```python
from build123d import *

# Parameters (mm, degrees)
F_1P5MM_64_START              = -32
F_1P5MM_64_DEPTH              = 64
CUT_EXTRUDE_M3_1_DEPTH        = 100
CUT_EXTRUDE_M3_1_DEPTH_BACK   = 100
SKETCH_2_R                    = 1.65
CUT_EXTRUDE_M3_1_2_DEPTH      = 100
CUT_EXTRUDE_M3_1_2_DEPTH_BACK = 100
SKETCH_3_R                    = 1.65
CUT_EXTRUDE_M3_1_3_DEPTH      = 100
CUT_EXTRUDE_M3_1_3_DEPTH_BACK = 100
SKETCH_4_R                    = 1.65
CUT_EXTRUDE_M3_1_4_DEPTH      = 100
CUT_EXTRUDE_M3_1_4_DEPTH_BACK = 100
SKETCH_5_R                    = 1.65


with BuildPart() as part:
    # 草图1 → 1p5mm铝合金直角座_宽64 (new body)
    with BuildSketch(Plane.XY.offset(F_1P5MM_64_START)):
        Polygon((0, 0), (16, 0), (16, 1.5), (1.5, 1.5), (1.5, 14), (0, 14), align=None)
    extrude(amount=F_1P5MM_64_DEPTH)

    # 草图2 → Cut-Extrude M3_-1 (cut, two sides: drawn at the far end of the back side and taken through both)
    with BuildSketch(Plane(origin=(0, 0, 0), x_dir=(0, 0, -1), z_dir=(1, 0, 0)).offset(-CUT_EXTRUDE_M3_1_DEPTH_BACK)):
        with Locations((24, 10)):
            Circle(SKETCH_2_R)
    extrude(amount=CUT_EXTRUDE_M3_1_DEPTH + CUT_EXTRUDE_M3_1_DEPTH_BACK, mode=Mode.SUBTRACT)

    # 草图3 → Cut-Extrude M3_-1 2 (cut, two sides: drawn at the far end of the back side and taken through both)
    with BuildSketch(Plane(origin=(0, 0, 0), x_dir=(1, 0, 0), z_dir=(0, 1, 0)).offset(-CUT_EXTRUDE_M3_1_2_DEPTH_BACK)):
        with Locations(Location((4.5, 22, 0), (0, 0, 270))):
            Circle(SKETCH_3_R)
    extrude(amount=CUT_EXTRUDE_M3_1_2_DEPTH + CUT_EXTRUDE_M3_1_2_DEPTH_BACK, mode=Mode.SUBTRACT)

    # 草图4 → Cut-Extrude M3_1 3 (cut, two sides: drawn at the far end of the back side and taken through both)
    with BuildSketch(Plane(origin=(0, 0, 0), x_dir=(0, 0, -1), z_dir=(1, 0, 0)).offset(-CUT_EXTRUDE_M3_1_3_DEPTH_BACK)):
        with Locations((-24, 10)):
            Circle(SKETCH_4_R)
    extrude(amount=CUT_EXTRUDE_M3_1_3_DEPTH + CUT_EXTRUDE_M3_1_3_DEPTH_BACK, mode=Mode.SUBTRACT)

    # 草图5 → Cut-Extrude M3_1 4 (cut, two sides: drawn at the far end of the back side and taken through both)
    with BuildSketch(Plane(origin=(0, 0, 0), x_dir=(1, 0, 0), z_dir=(0, 1, 0)).offset(-CUT_EXTRUDE_M3_1_4_DEPTH_BACK)):
        with Locations(Location((4.5, -22, 0), (0, 0, 270))):
            Circle(SKETCH_5_R)
    extrude(amount=CUT_EXTRUDE_M3_1_4_DEPTH + CUT_EXTRUDE_M3_1_4_DEPTH_BACK, mode=Mode.SUBTRACT)


solid = part.part
```
The listing builds one solid part. Answer for the finished solid, in the listing's coordinates (mm). A direction names the side the tool comes from. Give positions to 0.01 mm unless a question says otherwise; leave off trailing zeros. Write each loop counter-clockwise with the first axis right and the second up, starting at its lowest first coordinate (ties: lowest second). Pieces come first, ordered by that corner, then holes. Notation, with made-up numbers: (-34.5, -4.5) -> (-22.5, -4.5) arc R6 cw to (-22.5, -0.5) -> close; hole circle Ø10 at (2, -9). An arc over 180 degrees is marked (long way). Write item = value, one per line. Start each with the question number.
1) The part is cut by section B-B, the plane z = 16.5. Determine the outline of the cut face in (x, y), and give its area (4 significant figures).
2) The part is cut by section D-D, the plane x = 11. Determine the outline of the cut face in (y, z), and give its area (3 significant figures).
3) Each of these flat-tipped pins is pushed along its axis until it touches: pin 1 (8 mm diameter, centred on x = 8.5, z = -25.5, fed in from -Y); pin 2 (6 mm diameter, centred on y = 5, z = 2, fed in from +X); pin 3 (2.5 mm diameter, centred on y = 10, z = 24, fed in from -X); pin 4 (1.5 mm diameter, centred on x = 3, z = 0, fed in from +Y). Where does it stop, or does it pass through?
4) The part is cut by section C-C, the plane z = -21. Determine the outline of the cut face in (x, y).
5) Straight lines are drawn through the part: line 1 along Z through (x, y) = (0.4, 10); line 2 along Z through (x, y) = (4.5, 0.7); line 3 along Y through (x, z) = (0.3, 24). For each, find the intervals that lie inside material, in ascending order.
6) The part is cut by section A-A, the plane y = 10. Determine the outline of the cut face in (x, z).
7) Determine the mould class of faces 1 (the face through (0.74, 9, 25.31)), 2 (the face through (16, 1, 0)), 3 (the face through (9, 1.5, 0)) for opening direction Y: +Y half, -Y half, draft (parallel to the pull), parting line (faces both ways), or undercut.
8) Which of the six approach directions +Z, -Z, +X, -X, +Y, -Y give full straight-line access (tool end or side, diameter ignored) to faces 4 (the face through (4, 1, -32)), 5 (the face through (1.5, 8, 0))?
Solutions:
q1.outline = (0, 0) -> (16, 0) -> (16, 1.5) -> (1.5, 1.5) -> (1.5, 14) -> (0, 14) -> close
q1.area = 42.75 mm²
q2.outline = (0, -32) -> (1.5, -32) -> (1.5, 32) -> (0, 32) -> close
q2.area = 96.0 mm²
q3.pin_1 = 0
q3.pin_2 = 1.5
q3.pin_3 = through
q3.pin_4 = 1.5
q4.outline = (0, 0) -> (3.19, 0) -> (3.19, 1.5) -> (1.5, 1.5) -> (1.5, 14) -> (0, 14) -> close; (5.81, 0) -> (16, 0) -> (16, 1.5) -> (5.81, 1.5) -> close
q5.line_1 = -32 to -25.65, -22.35 to 22.35, 25.65 to 32
q5.line_2 = -32 to -23.65, -20.35 to 20.35, 23.65 to 32
q5.line_3 = 0 to 8.35, 11.65 to 14
q6.outline = (0, -32) -> (1.5, -32) -> (1.5, -25.65) -> (0, -25.65) -> close; (0, -22.35) -> (1.5, -22.35) -> (1.5, 22.35) -> (0, 22.35) -> close; (0, 25.65) -> (1.5, 25.65) -> (1.5, 32) -> (0, 32) -> close
q7.face_1 = undercut
q7.face_2 = draft
q7.face_3 = +Y half
q8.face_4 = -Z, +X, -X, +Y, -Y
q8.face_5 = +Z, -Z, +X, +Y
